```python
from build123d import *
from build123d.topology import SkipClean

# Parameters (mm, degrees)
BOSS_EXTRUDE1_DEPTH  = 20
SKETCH2_W            = 60
SKETCH2_H            = 20
CUT_EXTRUDE1_DEPTH   = 20
FILLET1_R            = 9.75
FILLET1_OF_MIRROR4_R = 9.75
SKETCH4_R            = 2.1
CUT_EXTRUDE3_DEPTH   = 20


with BuildPart() as part:
    # Sketch1 → Boss-Extrude1 (new body)
    with BuildSketch(Plane(origin=(0, 0, 0), x_dir=(1, 0, 0), z_dir=(0, 1, 0))):
        with BuildLine():
            Line((22.360679775, 20), (90, 20))
            Line((90, 20), (90, -20))
            Line((90, -20), (22.360679775, -20))
            ThreePointArc((22.360679775, -20), (12.247448714, -27.386127875), (0, -30))
            Line((0, -30), (0, -20))
            Line((0, -20), (0, 20))
            Line((0, 20), (0, 30))
            ThreePointArc((0, 30), (12.247448714, 27.386127875), (22.360679775, 20))
        make_face()
    boss_extrude1 = extrude(amount=BOSS_EXTRUDE1_DEPTH)

    # Sketch2 → Cut-Extrude1 (cut)
    with BuildSketch(Plane(origin=(0, 20, 0), x_dir=(1, 0, 0), z_dir=(0, 1, 0))):
        with BuildLine():
            Line((0, 6.3), (0, -6.3))
            ThreePointArc((0, -6.3), (6.3, 0), (0, 6.3))
        make_face()
        with Locations((60, 0)):
            Rectangle(SKETCH2_W, SKETCH2_H)
    cut_extrude1 = extrude(amount=-CUT_EXTRUDE1_DEPTH, mode=Mode.SUBTRACT)

    # Fillet1
    fillet1_edges = [part.edges().sort_by_distance(p)[0] for p in [
        (90, 10, -20),
        (90, 10, 20),
    ]]
    fillet(fillet1_edges, radius=FILLET1_R)

    # Mirror4: Boss-Extrude1, Cut-Extrude1 across plane
    with SkipClean():  # the faces are left unmerged after this step: merging them gives an invalid solid
        add(boss_extrude1.mirror(Plane(origin=(0, 0, 0), x_dir=(0, 0, 1), z_dir=(1, 0, 0))))
        add(cut_extrude1.mirror(Plane(origin=(0, 0, 0), x_dir=(0, 0, 1), z_dir=(1, 0, 0))), mode=Mode.SUBTRACT)
    add(part.part.scale(1), mode=Mode.REPLACE)  # the faces are merged on a copy

    # Fillet1 of Mirror4
    fillet1_of_mirror4_edges = [part.edges().sort_by_distance(p)[0] for p in [
        (-90, 10, -20),
        (-90, 10, 20),
    ]]
    fillet(fillet1_of_mirror4_edges, radius=FILLET1_OF_MIRROR4_R)

    # Sketch4 → Cut-Extrude3 (cut)
    with BuildSketch(Plane(origin=(0, 20, 0), x_dir=(1, 0, 0), z_dir=(0, 1, 0))):
        with Locations(Location((21, 0, 0), (0, 0, 270))):
            Circle(SKETCH4_R)
        with Locations(Location((14.849242405, -14.849242405, 0), (0, 0, 270))):
            Circle(SKETCH4_R)
        with Locations(Location((0, -21, 0), (0, 0, 270))):
            Circle(SKETCH4_R)
        with Locations(Location((-14.849242405, -14.849242405, 0), (0, 0, 270))):
            Circle(SKETCH4_R)
        with Locations(Location((-21, 0, 0), (0, 0, 270))):
            Circle(SKETCH4_R)
        with Locations(Location((-14.849242405, 14.849242405, 0), (0, 0, 270))):
            Circle(SKETCH4_R)
        with Locations(Location((0, 21, 0), (0, 0, 270))):
            Circle(SKETCH4_R)
        with Locations(Location((14.849242405, 14.849242405, 0), (0, 0, 270))):
            Circle(SKETCH4_R)
    extrude(amount=-CUT_EXTRUDE3_DEPTH, mode=Mode.SUBTRACT)


solid = part.part
```
Source: CAD feature listing. Evaluate the final solid. Frame: model axes, mm. A direction names the side the tool comes from. Coordinates: 2 decimals unless noted, no trailing zeros. Write each loop counter-clockwise with the first axis right and the second up, starting at its lowest first coordinate (ties: lowest second). Pieces come first, ordered by that corner, then holes. Notation, with made-up numbers: (23.25, 47) - (59.25, 47) arc R14 cw to (59.25, 64) - close; hole circle Ø3 at (78, 4). An arc over 180 degrees is marked (long way). Answer as a JSON object with one key per item and string values.
Q1. Section query C-C, the plane z = 0. Output: boundary loops of the cut face in (x, y).
Ans:
{"outline": "(-30, 0) - (-23.1, 0) - (-23.1, 20) - (-30, 20) - close; (-18.9, 0) - (-6.3, 0) - (-6.3, 20) - (-18.9, 20) - close; (6.3, 0) - (18.9, 0) - (18.9, 20) - (6.3, 20) - close; (23.1, 0) - (30, 0) - (30, 20) - (23.1, 20) - close"}
Q2. Draft query along Z for faces 1 (the cylindrical face through (-12.767, 10.14, 14.576)), 2 (the cylindrical face through (22.77, 10.14, 1.13)), 3 (the cylindrical face through (-87.07, 10.14, -17.22)), 4 (the cylindrical face through (87.07, 10.14, 17.22)). Return one class per face: released by +Z, released by -Z, zero draft, split by the parting line, or undercut.
Ans:
{"face 1": "undercut", "face 2": "undercut", "face 3": "released by -Z", "face 4": "released by +Z"}
Q3. Section query B-B, the plane z = 15. Output: boundary loops of the cut face in (x, y).
Ans:
{"outline": "(-88.76, 0) - (-16.94, 0) - (-16.94, 20) - (-88.76, 20) - close; (-12.75, 0) - (12.75, 0) - (12.75, 20) - (-12.75, 20) - close; (16.94, 0) - (88.76, 0) - (88.76, 20) - (16.94, 20) - close"}
Q4. Section query D-D, the plane y = 5.5. State how many separate pieces and enclosed holes the cut face has, plus the area to 3 significant figures.
Ans:
{"separate pieces": "1", "enclosed holes": "9", "area": "5,100 mm2"}
Q5. First-contact query: pin 1 Ø1.5 at (x, z) = (-12.5, 18.5) entering from -Y; pin 2 Ø10 at (x, y) = (-63.5, 13.5) entering from -Z; pin 3 Ø3 at (y, z) = (14.5, 23) entering from -X; pin 4 Ø3 at (x, y) = (-13.5, 18) entering from -Z. Flat tips, straight axial feed; report the tip coordinate or a pass-through.
Ans:
{"pin 1": "stops at y = 0", "pin 2": "stops at z = -20", "pin 3": "stops at x = -20.92", "pin 4": "stops at z = -27.5"}
Q6. Material intervals for line 1 (X direction, y = 14.5, z = 0); line 2 (Z direction, x = 62, y = 11.25); line 3 (X direction, y = 6, z = 15.5), sorted ascending. Write a range as [from, to].
Ans:
{"line 1": "x = [-30, -23.1], [-18.9, -6.3], [6.3, 18.9], [23.1, 30]", "line 2": "z = [-20, -10], [10, 20]", "line 3": "x = [-88.47, -16.85], [-12.85, 12.85], [16.85, 88.47]"}
Q7. Section query A-A, the plane x = -46. Output: boundary loops of the cut face in (y, z).
Ans:
{"outline": "(0, -20) - (20, -20) - (20, -10) - (0, -10) - close; (0, 10) - (20, 10) - (20, 20) - (0, 20) - close"}
Q8. Set-up query: faces 5 (the flat face through (-52, 10, 20)), 6 (the flat face through (60, 10, -10)), 7 (the flat face through (-60, 10, -10)), 8 (the flat face through (-51, 10, -20)). Return all of +Z, -Z, +X, -X, +Y, -Y with unobstructed straight access to the full face (end or side cutting, diameter ignored); none if empty.
Ans:
{"face 5": "+Z, -X, +Y, -Y", "face 6": "+X, +Y, -Y", "face 7": "-X, +Y, -Y", "face 8": "-Z, -X, +Y, -Y"}
